For this review, take the finished solid that the model builds, in its own axes (mm). A direction names the side the tool comes from. Round coordinates to 2 decimals unless told otherwise and drop trailing zeros.
```python
from build123d import *

# Parameters (mm, degrees)
BOSS_EXTRUDE2_DEPTH = 3
FILLET1_R           = 10


with BuildPart() as part:
    # Sketch1 → Boss-Extrude2 (new body)
    with BuildSketch(Plane(origin=(0, 0, 0), x_dir=(1, 0, 0), z_dir=(0, 1, 0))):
        with BuildLine():
            Line((83.277636848, 6.577391731), (36.063202158, -10.996818305))
            ThreePointArc((36.063202158, -10.996818305), (32.802532832, -11.889585683), (29.435258028, -12.19034879))
            Line((29.435258028, -12.19034879), (13.331621464, -12.19034879))
            ThreePointArc((13.331621464, -12.19034879), (11.631621464, -13.89034879), (13.331621464, -15.59034879))
            Line((13.331621464, -15.59034879), (31.335553361, -15.59034879))
            ThreePointArc((31.335553361, -15.59034879), (32.329091164, -24.600925987), (31.335553361, -33.611503185))
            Line((31.335553361, -33.611503185), (5.718159441, -30.692769825))
            ThreePointArc((5.718159441, -30.692769825), (3.836641823, -32.189396516), (5.333268515, -34.070914135))
            Line((5.333268515, -34.070914135), (32.258758745, -37.138686243))
            ThreePointArc((32.258758745, -37.138686243), (30.141236011, -41.228168064), (25.83833159, -42.869136571))
            Line((25.83833159, -42.869136571), (3.931607644, -43.234741077))
            Line((3.931607644, -43.234741077), (1.645004408, -44.879459267))
            ThreePointArc((1.645004408, -44.879459267), (-0.44755249, -45.424610965), (-2.363050322, -44.421190413))
            ThreePointArc((-2.363050322, -44.421190413), (-16.657617756, -35.649988568), (-33.406545395, -36.511419261))
            ThreePointArc((-33.406545395, -36.511419261), (-35.065515769, -36.818007167), (-36.732015424, -36.555409102))
            Line((-36.732015424, -36.555409102), (-43.072013441, -34.41346595))
            ThreePointArc((-43.072013441, -34.41346595), (-44.756883472, -34.602804193), (-45.690953078, -36.017777677))
            ThreePointArc((-45.690953078, -36.017777677), (-44.377060251, -43.944176391), (-38.701961301, -49.631650596))
            ThreePointArc((-38.701961301, -49.631650596), (-48.89375638, -45.294039559), (-53.199015105, -35.088535957))
            ThreePointArc((-53.199015105, -35.088535957), (-57.963880411, -31.924307539), (-60.880420097, -27.003933658))
            ThreePointArc((-60.880420097, -27.003933658), (-60.719986784, -25.061085947), (-59.232742508, -23.80072864))
            ThreePointArc((-59.232742508, -23.80072864), (-56.720776297, -23.205324241), (-54.14697512, -23.005253893))
            ThreePointArc((-54.14697512, -23.005253893), (-52.817288904, -22.454479829), (-52.26651484, -21.124793613))
            Line((-52.26651484, -21.124793613), (-52.26651484, -18.255253893))
            ThreePointArc((-52.26651484, -18.255253893), (-51.768596368, -17.053172365), (-50.56651484, -16.555253893))
            Line((-50.56651484, -16.555253893), (-50.18504008, -16.555253893))
            Line((-50.18504008, -16.555253893), (-50.18504008, -21.008976099))
            ThreePointArc((-50.18504008, -21.008976099), (-49.292805972, -23.163019785), (-47.138762286, -24.055253893))
            Line((-47.138762286, -24.055253893), (-38.258057554, -24.055253893))
            ThreePointArc((-38.258057554, -24.055253893), (-32.429820226, -23.139270307), (-27.163537606, -20.479638066))
            Line((-27.163537606, -20.479638066), (-18.213895237, -14.042299326))
            ThreePointArc((-18.213895237, -14.042299326), (-17.803794916, -13.348327859), (-18.036830501, -12.576658832))
            ThreePointArc((-18.036830501, -12.576658832), (-21.621060958, -9.471725354), (-25.963310125, -7.565894288))
            Line((-25.963310125, -7.565894288), (-55.30954126, 0.349304832))
            ThreePointArc((-55.30954126, 0.349304832), (-56.903028243, 0.142191478), (-57.883342437, -1.131025232))
            Line((-57.883342437, -1.131025232), (-57.883342437, -6.467193959))
            Line((-57.883342437, -6.467193959), (-59.970418868, -6.467193959))
            ThreePointArc((-59.970418868, -6.467193959), (-62.745333472, -5.626502668), (-64.58710946, -3.387133535))
            ThreePointArc((-64.58710946, -3.387133535), (-65.510981808, 5.487804074), (-61.413967112, 13.414501258))
            ThreePointArc((-61.413967112, 13.414501258), (-58.998069827, 14.801189981), (-56.215124926, 14.680016601))
            Line((-56.215124926, 14.680016601), (-13.213967112, 0.152246204))
            Line((-13.213967112, 0.152246204), (-13.195522989, -7.843254171))
            ThreePointArc((-13.195522989, -7.843254171), (-11.391375526, -9.63909713), (-9.595532567, -7.834949667))
            Line((-9.595532567, -7.834949667), (-9.645178165, 13.686344484))
            Line((-9.645178165, 13.686344484), (3.240530108, 9.701083124))
            add(Edge.make_bspline(
                [(3.240530108, 9.701083124), (13.894797432, -10.964082924), (52.167573777, 8.768078407), (90.440350123, 28.500239738), (79.7860828, 49.165405786)],
                knots=[0, 0, 0, 1.570796327, 1.570796327, 3.141592654, 3.141592654, 3.141592654], degree=2, weights=[1, 0.707106781, 1, 0.707106781, 1]))
            ThreePointArc((79.7860828, 49.165405786), (80.072864648, 50.071466121), (80.980537261, 49.789828788))
            ThreePointArc((80.980537261, 49.789828788), (84.258913327, 36.167877688), (80.573020022, 22.650500281))
            ThreePointArc((80.573020022, 22.650500281), (80.977131886, 20.603840239), (83.060820169, 20.705658035))
            ThreePointArc((83.060820169, 20.705658035), (96.799731472, 40.905147255), (100.995247842, 64.971195766))
            ThreePointArc((100.995247842, 64.971195766), (102.023911204, 66.136579392), (103.234366802, 65.161354006))
            ThreePointArc((103.234366802, 65.161354006), (102.922479327, 43.72601882), (96.524889391, 23.265282974))
            ThreePointArc((96.524889391, 23.265282974), (96.918331366, 21.170533694), (99.034577715, 20.917013432))
            ThreePointArc((99.034577715, 20.917013432), (110.533106389, 30.95950626), (117.098161764, 44.742389549))
            ThreePointArc((117.098161764, 44.742389549), (118.133339849, 45.458434414), (118.968319872, 44.516562727))
            ThreePointArc((118.968319872, 44.516562727), (109.903683893, 20.121141501), (87.108506166, 7.563909538))
            ThreePointArc((87.108506166, 7.563909538), (85.167327095, 7.170621945), (83.277636848, 6.577391731))
        make_face()
    extrude(amount=BOSS_EXTRUDE2_DEPTH)

    # Fillet1
    fillet1_edges = [part.edges().sort_by_distance(p)[0] for p in [
        (3.240530108, 1.5, -9.701083124),
    ]]
    fillet(fillet1_edges, radius=FILLET1_R)


solid = part.part
```
Q1. Mouldability with a two-part tool opening along X and no side actions: class faces 6 (the face through (110.145, 1.479, -20.404)), 7 (the face through (102.97, 1.48, -44.02)), 8 (the face through (-48.781, 1.479, 45.406)) as +X half, -X half, draft (parallel to the pull), parting line (faces both ways), or undercut.
Q2. Wall thickness on line 1 (X direction, y = 0.8, z = -39); line 2 (X direction, y = 2.75, z = -43); line 3 (Z direction, x = 27, y = 0.35): over which ranges is each line inside the solid? List them lowest first.
Q3. Clearance check with flat-ended pins moving along their axes: pin 1 (1 mm diameter, centred on x = 50.5, y = 1, fed in from +Z); pin 2 (0.6 mm diameter, centred on x = -59.5, y = 1.5, fed in from +Z); pin 3 (0.9 mm diameter, centred on x = -44, y = 1, fed in from -Z). State where each tip first meets the part, or that it passes through.
Q4. Take a section at A-A, the plane z = -28. Count the separate pieces of the cut face and the enclosed holes in it, plus the area to 3 significant figures.
Q5. Tool access review of faces 1 (the face through (-35.02, 1.48, -7.52)), 2 (the face through (30.19, 1.479, 41.184)), 3 (the face through (84.26, 1.48, -36.37)), 4 (the face through (-57.91, 1.48, 31.98)), 5 (the face through (-21.56, 1.48, 9.51)): name each direction out of +Z, -Z, +X, -X, +Y, -Y from which nothing blocks a thin tool from reaching the whole face with its end or side.
Working result:
1. face 6: +X half
1. face 7: undercut
1. face 8: -X half
2. line 1: x = 80.8 to 84.16, 95.99 to 102.01, 115.19 to 118.56
2. line 2: x = 81.24 to 83.52, 97.6 to 102.8, 116.63 to 118.94
2. line 3: z = -1.06 to 12.19, 15.59 to 33.12, 36.54 to 42.76
3. pin 1: stops at z = 5.81
3. pin 2: stops at z = 30.41
3. pin 3: stops at z = -10.71
4. separate pieces: 3
4. enclosed holes: 0
4. area: 70.5 mm2
5. face 1: -Z, +Y, -Y
5. face 2: +Z, +X, +Y, -Y
5. face 3: +Y, -Y
5. face 4: +Z, -X, +Y, -Y
5. face 5: -X, +Y, -Y
